```python
from build123d import *

# Parameters (mm, degrees)
SKETCH1_W           = 838.2
SKETCH1_H           = 757.2375
BOSS_EXTRUDE1_DEPTH = 19.05
CUT_EXTRUDE1_DEPTH  = 839.2


with BuildPart() as part:
    # Sketch1 → Boss-Extrude1 (new body)
    with BuildSketch(Plane(origin=(0, 0, 0), x_dir=(1, 0, 0), z_dir=(0, 1, 0))):
        with Locations((419.1, 378.61875)):
            Rectangle(SKETCH1_W, SKETCH1_H)
    extrude(amount=BOSS_EXTRUDE1_DEPTH)

    # Sketch3 → Cut-Extrude1 (cut, through all)
    with BuildSketch(Plane(origin=(838.2, 0, 0), x_dir=(0, 0, -1), z_dir=(1, 0, 0))):
        Polygon((421.17645, 0), (421.17645, 5.96265), (423.84345, 5.96265), (423.84345, 9.51865), (399.45945, 9.51865), (399.45945, 5.96265), (402.12645, 5.96265), (402.12645, 0), align=None)
    extrude(amount=-CUT_EXTRUDE1_DEPTH, mode=Mode.SUBTRACT)


solid = part.part
```
For this review, take the finished solid that the model builds, in its own axes (mm). Coordinates: 2 decimals unless noted, no trailing zeros. Answer as a JSON object with one key per item and string values. Group by question number.
1. Clearance check with a flat-ended pin moving along its axis: P1, Ø7.5, axis at x = 306.5, z = -410, coming from the -Y side. State where the tip first meets the part, or that it passes through.
2. The part is to be moulded in two halves that separate along Z. For faces 1 (the flat face through (413, 9, 0)), 2 (the flat face through (413, 0, -204)), 3 (the flat face through (425, 9.519, -412)), say which applies: pulls with the +Z half, pulls with the -Z half, needs draft (parallel to the pull), parting line crosses it, or undercut.
3. For probe 1 along Z at (x, y) = (804, 2); probe 2 along Z at (x, y) = (94, 8), list the stretches that pass through material, from the lowest coordinate up.
Final values:
{
 "1": {"P1": "y = 9.52"},
 "2": {"face 1": "pulls with the +Z half", "face 2": "needs draft", "face 3": "undercut"},
 "3": {"probe 1": "-757.24 to -421.18, -402.13 to 0", "probe 2": "-757.24 to -423.84, -399.46 to 0"}
}
